```python
from build123d import *

# Parameters (mm, degrees)
F0_R     = 12.7
F1_DEPTH = 38.1
F2_R     = 6.35
F3_DEPTH = 25.4


with BuildPart() as f1:
    # F0 (on Front) → F1 (new body)
    with BuildSketch(Plane.XZ):
        with BuildLine():
            Line((-103.032803, -9.998872), (23.967197, -9.998872))
            Line((23.967197, -9.998872), (23.967197, 2.701128))
            Line((23.967197, 2.701128), (-6.750105, 2.701128))
            ThreePointArc((-6.750105, 2.701128), (-15.802905, 8.10209), (-20.597679, 17.490047))
            ThreePointArc((-20.597679, 17.490047), (-20.730839, 18.259479), (-20.832355, 19.03372))
            ThreePointArc((-20.832355, 19.03372), (-39.532803, 34.451128), (-58.233251, 19.03372))
            ThreePointArc((-58.233251, 19.03372), (-58.334767, 18.259479), (-58.467927, 17.490047))
            ThreePointArc((-58.467927, 17.490047), (-63.262701, 8.10209), (-72.315501, 2.701128))
            Line((-72.315501, 2.701128), (-103.032803, 2.701128))
            Line((-103.032803, 2.701128), (-103.032803, -9.998872))
        make_face()
        with Locations((-39.532803, 15.401128)):
            Circle(F0_R, mode=Mode.SUBTRACT)
        with BuildLine():
            ThreePointArc((-20.832355, 19.03372), (-20.730839, 18.259479), (-20.597679, 17.490047))
            ThreePointArc((-20.597679, 17.490047), (-20.699195, 18.264289), (-20.832355, 19.03372))
        make_face()
        with BuildLine():
            ThreePointArc((-58.233251, 19.03372), (-58.366411, 18.264289), (-58.467927, 17.490047))
            ThreePointArc((-58.467927, 17.490047), (-58.334767, 18.259479), (-58.233251, 19.03372))
        make_face()
    extrude(amount=F1_DEPTH)

    # F2 (on face) → F3 (cut)
    with BuildSketch(Plane.XY.offset(2.701128)):
        with Locations((-83.982803, -19.05)):
            Circle(F2_R)
        with Locations((4.917197, -19.05)):
            Circle(F2_R)
    extrude(amount=-F3_DEPTH, mode=Mode.SUBTRACT)


solid = f1.part
```
Geometry: final body of the model. Coordinates: model frame, mm. A direction names the side the tool comes from. Coordinates: 2 decimals unless noted, no trailing zeros. Order: outer loops, then holes, each group sorted by start corner. A loop starts at its lowest first (then second) coordinate and runs counter-clockwise, first axis right, second up. Notation, with made-up numbers: (41, -33.75) -> (50, -33.75) arc R16 ccw to (50, -16.75) -> close; hole circle Ø5 at (-25.5, 37). An arc over 180 degrees is marked (long way). Write each question's results on one line, items separated by ' | '. Start each with the question number.
1) Cut plane B-B, the plane z = -7. Output: boundary loops of the cut face in (x, y).
2) Cut plane D-D, the plane x = 0. Output: boundary loops of the cut face in (y, z).
3) Cut plane C-C, the plane y = -33.5. Output: boundary loops of the cut face in (x, z).
4) Set-up query: faces 1 (the flat face through (-40, -38.1, -2)), 2 (the flat face through (-91, -19, 2.701)). Return all of +Z, -Z, +X, -X, +Y, -Y with unobstructed straight access to the full face (end or side cutting, diameter ignored); none if empty.
5) Cut plane A-A, the plane y = -16. Output: boundary loops of the cut face in (x, z), and give its area (3 significant figures).
6) First-contact query: pin 1 (14.5 mm diameter, centred on x = 4.92, y = -19.05, fed in from +Z); pin 2 (11.5 mm diameter, centred on x = -83.98, y = -19.05, fed in from -Z); pin 3 (8 mm diameter, centred on y = -11, z = 12, fed in from -X); pin 4 (1.5 mm diameter, centred on y = -18.5, z = 6.5, fed in from -X). Flat tips, straight axial feed; report the tip coordinate or a pass-through.
7) Mould query, pull axis Z, two halves, no side actions, for faces 3 (the cylindrical face through (-90.327, -18.771, -3.56)), 4 (the cylindrical face through (-49.61, -18.78, 7.67)), 5 (the flat face through (12, -19, 2.701)). Classes: released by +Z, released by -Z, zero draft, split by the parting line, or undercut.
8) Material intervals for line 1 along X through (y, z) = (-19, -2); line 2 along Z through (x, y) = (-82.5, -7); line 3 along Z through (x, y) = (-44.5, -10), sorted ascending.
Checks:
1) outline: (-103.03, -38.1) -> (23.97, -38.1) -> (23.97, 0) -> (-103.03, 0) -> close; hole circle Ø12.7 at (-83.98, -19.05); hole circle Ø12.7 at (4.92, -19.05)
2) outline: (-38.1, -10) -> (-23.07, -10) -> (-23.07, 2.7) -> (-38.1, 2.7) -> close; (-15.03, -10) -> (0, -10) -> (0, 2.7) -> (-15.03, 2.7) -> close
3) outline: (-103.03, -10) -> (23.97, -10) -> (23.97, 2.7) -> (-6.75, 2.7) arc R19.05 cw to (-20.6, 17.49) arc R19.05 ccw to (-20.83, 19.03) arc R19.05 ccw to (-58.23, 19.03) arc R19.05 ccw to (-58.47, 17.49) arc R19.05 cw to (-72.32, 2.7) -> (-103.03, 2.7) -> close; hole circle Ø25.4 at (-39.53, 15.4)
4) face 1: +Z, -Z, +X, -X, -Y | face 2: +Z, -X, +Y, -Y
5) outline: (-103.03, -10) -> (-89.55, -10) -> (-89.55, 2.7) -> (-103.03, 2.7) -> close; (-78.41, -10) -> (-0.65, -10) -> (-0.65, 2.7) -> (-6.75, 2.7) arc R19.05 cw to (-20.6, 17.49) arc R19.05 ccw to (-20.83, 19.03) arc R19.05 ccw to (-58.23, 19.03) arc R19.05 ccw to (-58.47, 17.49) arc R19.05 cw to (-72.32, 2.7) -> (-78.41, 2.7) -> close; (10.49, -10) -> (23.97, -10) -> (23.97, 2.7) -> (10.49, 2.7) -> close; hole circle Ø25.4 at (-39.53, 15.4) | area: 2,000 mm^2
6) pin 1: z = 2.7 | pin 2: through | pin 3: x = -63.36 | pin 4: x = -65.92
7) face 3: zero draft | face 4: undercut | face 5: released by +Z
8) line 1: -103.03 to -90.33, -77.63 to -1.43, 11.27 to 23.97 | line 2: -10 to 2.7 | line 3: -10 to 3.71, 27.09 to 33.79
